from build123d import *

# Parameters (mm, degrees)
SKETCH_1_W          = 20
SKETCH_1_H          = 10.5
EXTRUDE_1_DEPTH     = 6.5
SKETCH_2_R          = 1.25
CUT_EXTRUDE_1_DEPTH = 6.5
SKETCH_3_W          = 4.44626532
SKETCH_3_H          = 1.008872475
SKETCH_3_W_2        = 5
SKETCH_3_W_3        = 3.65317203
CUT_EXTRUDE_2_DEPTH = 6.5
CHAMFER_1_SIZE      = 0.45
SKETCH_4_W          = 10.31021277
SKETCH_4_H          = 1.008783122
CUT_EXTRUDE_3_DEPTH = 6.5
CHAMFER_2_SIZE      = 0.75
EXTRUDE_2_DEPTH     = 4


with BuildPart() as part:
    # 스케치1 → 보스-돌출1 (new body)
    with BuildSketch(Plane(origin=(0, 0, 0), x_dir=(1, 0, 0), z_dir=(0, 1, 0))):
        Rectangle(SKETCH_1_W, SKETCH_1_H)
    extrude(amount=EXTRUDE_1_DEPTH)

    # 스케치2 → 컷-돌출1 (cut)
    with BuildSketch(Plane(origin=(0, 6.5, 0), x_dir=(1, 0, 0), z_dir=(0, 1, 0))):
        with Locations(Location((-4.75, -2.1, 0), (0, 0, 270))):
            Circle(SKETCH_2_R)
        with Locations(Location((4.75, -2.1, 0), (0, 0, 270))):
            Circle(SKETCH_2_R)
    extrude(amount=-CUT_EXTRUDE_1_DEPTH, mode=Mode.SUBTRACT)

    # 스케치3 → 컷-돌출2 (cut)
    with BuildSketch(Plane(origin=(0, 6.5, 0), x_dir=(1, 0, 0), z_dir=(0, 1, 0))):
        with Locations((-9.22313266, -5.304436238)):
            Rectangle(SKETCH_3_W, SKETCH_3_H)
        with Locations((0, -5.304436238)):
            Rectangle(SKETCH_3_W_2, SKETCH_3_H)
        with Locations((8.826586015, -5.304436238)):
            Rectangle(SKETCH_3_W_3, SKETCH_3_H)
    extrude(amount=-CUT_EXTRUDE_2_DEPTH, mode=Mode.SUBTRACT)

    # 모따기1
    chamfer_1_edges = [part.edges().sort_by_distance(p)[0] for p in [
        (7, 3.25, 5.25),
        (2.5, 3.25, 5.25),
        (-2.5, 3.25, 5.25),
        (-7, 3.25, 5.25),
    ]]
    chamfer(chamfer_1_edges, length=CHAMFER_1_SIZE - 0.0001)  # a hair under: the kernel refuses the full size

    # 스케치4 → 컷-돌출3 (cut)
    with BuildSketch(Plane(origin=(0, 6.5, 0), x_dir=(1, 0, 0), z_dir=(0, 1, 0))):
        with Locations((5.155106385, 5.004391561)):
            Rectangle(SKETCH_4_W, SKETCH_4_H)
    extrude(amount=-CUT_EXTRUDE_3_DEPTH, mode=Mode.SUBTRACT)

    # 모따기2
    chamfer_2_edges = [part.edges().sort_by_distance(p)[0] for p in [
        (0, 3.25, -5.25),
    ]]
    chamfer(chamfer_2_edges, length=CHAMFER_2_SIZE - 0.0001)  # a hair under: the kernel refuses the full size

    # 스케치5 → 보스-돌출2 (add)
    with BuildSketch(Plane(origin=(0, 5.25, 0), x_dir=(1, 0, 0), z_dir=(0, 1, 0))):
        Polygon((-6.65, 5.25), (-7, 5.25), (-7, 5.807319656), (9.3, 9.495633097), (9.377244102, 9.154263285), (-6.65, 5.527668202), align=None)
    extrude(amount=-EXTRUDE_2_DEPTH)


solid = part.part
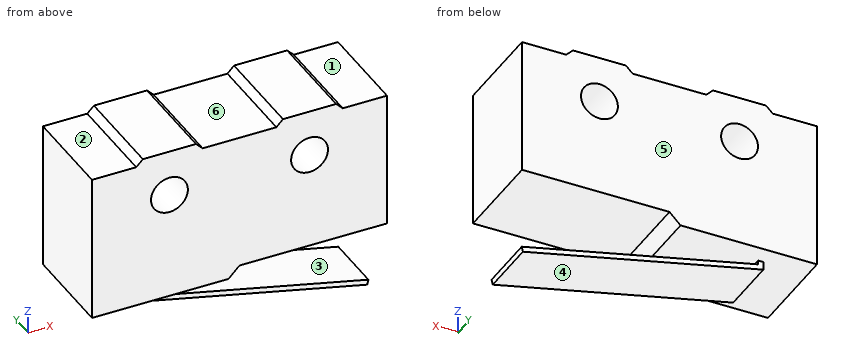
Read the model definition and answer for the solid it produces. Units are mm, in the model's axes. Face numbers are marked on the shaded views. A direction names the side the tool comes from. Give positions to 0.01 mm unless a question says otherwise; leave off trailing zeros. Loops run counter-clockwise (first coordinate to the right, second up) from the corner with the lowest first, then second, coordinate; pieces in that order, holes last. Notation, with made-up numbers: M -26.5,36 L -14.5,36 A35 cw -14.5,75 Z; hole C 5,85 d1. An arc over 180 degrees is marked long. Write each question's results on one line, items separated by ' | '.
1. Straight lines are drawn through the part: line 1 (X direction, y = 2.5, z = 2.1); line 2 (Z direction, x = -5.75, y = 3.5); line 3 (X direction, y = 0.5, z = 1.5). For each, find the intervals that lie inside material, in ascending order. Write a range as [from, to].
Values:
line 1: x = [-10, -6], [-3.5, 3.5], [6, 10] | line 2: z = [-6.09, -5.73], [-5.25, 1.35], [2.85, 5.25] | line 3: x = [-10, -5.85], [-3.65, 3.65], [5.85, 10]
2. The mould has two halves that part along X. Classify the marked faces 4, 5 and 6: pulls with the +X half, pulls with the -X half, needs draft (parallel to the pull), parting line crosses it, or undercut.
Values:
face 4: pulls with the -X half | face 5: needs draft | face 6: undercut
3. Section B-B on y = 4.5 is taken. State how many separate pieces and enclosed holes the cut face has, plus the area to 3 significant figures.
Values:
separate pieces: 1 | enclosed holes: 2 | area: 193 mm^2
4. Section D-D on x = 4.75 is taken. Give the vertices of the cut face in (y, z).
Values:
outline: M 0,-4.5 L 6.5,-4.5 L 6.5,0.85 L 0,0.85 Z; M 0,3.35 L 6.5,3.35 L 6.5,5.25 L 0,5.25 Z; M 1.25,-8.47 L 5.25,-8.47 L 5.25,-8.11 L 1.25,-8.11 Z
5. Section A-A on z = 1.75 is taken. Give the vertices of the cut face in (x, y), plus the area to 3 significant figures.
Values:
outline: M -10,0 L -5.95,0 L -5.95,6.5 L -10,6.5 Z; M -3.55,0 L 3.55,0 L 3.55,6.5 L -3.55,6.5 Z; M 5.95,0 L 10,0 L 10,6.5 L 5.95,6.5 Z | area: 98.8 mm^2
6. A tool of negligible diameter and unlimited length cuts with its end or side. For the marked faces 1, 2 and 3, from which of +Z, -Z, +X, -X, +Y, -Y can it reach the whole face along a straight path? Write none if from no direction.
Values:
face 1: +Z, +X, +Y, -Y | face 2: +Z, -X, +Y, -Y | face 3: +X, +Y, -Y
7. Section C-C on x = -1 is taken. Give the vertices of the cut face in (y, z).
Values:
outline: M 0,-5.25 L 6.5,-5.25 L 6.5,4.8 L 0,4.8 Z; M 1.25,-7.16 L 5.25,-7.16 L 5.25,-6.81 L 1.25,-6.81 Z
8. Given pin 1 (2 mm diameter, centred on x = 2.5, z = -7.5, fed in from +Y); pin 2 (2.5 mm diameter, centred on x = -8.5, y = 2.5, fed in from +Z), each flat-ended and moving along its own axis, determine where each tip first touches the part or whether it passes through.
Values:
pin 1: stops at y = 5.25 | pin 2: stops at z = 4.8
